Source: CAD feature listing. Evaluate the final solid. Frame: model axes, mm. Give positions to 0.01 mm unless a question says otherwise; leave off trailing zeros. Order: outer loops, then holes, each group sorted by start corner. A loop starts at its lowest first (then second) coordinate and runs counter-clockwise, first axis right, second up. Notation, with made-up numbers: M 84.5,-27 L 113.5,-27 A22 ccw 113.5,-6 Z; hole C 19.25,-34 d6. An arc over 180 degrees is marked long. Use CSV: the item, a comma, the result in double quotes. Start each with the question number.
Item 1: First-contact query: pin 1 (1 mm diameter, centred on x = -70, y = -2.5, fed in from +Z); pin 2 (1.2 mm diameter, centred on x = -100.5, y = -3, fed in from -Z). Flat tips, straight axial feed; report the tip coordinate or a pass-through.
Item 2: Ray query, probe 1 along Z at (x, y) = (-5, -1.45); probe 2 along Z at (x, y) = (47, -3.8); probe 3 along Z at (x, y) = (-62, -1.1). Return the intervals inside material, ascending. Write a range as from..to.
Item 3: Section query A-A on y = -3.1. Return loops of the section in (x, z), and give its area (3 significant figures).
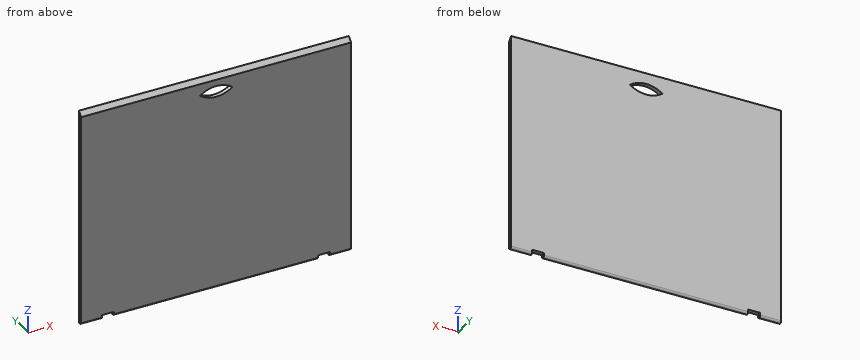
from build123d import *

# Parameters (mm, degrees)
F0_W     = 250
F0_H     = 197
F1_DEPTH = 4
F3_W     = 11
F3_H     = 4
F4_DEPTH = 0.5
F5_DEPTH = 250
F6_DEPTH = 25
F8_DEPTH = 25
F9_SIZE  = 3.99999


# Not quite as in the source:
# - a fillet or chamfer is up to 0.001 mm smaller than in the source, because OpenCascade refuses the exact size


with BuildPart() as f1:
    # F0 (on Front) → F1 (new body)
    with BuildSketch(Plane.XZ):
        Rectangle(F0_W, F0_H)
    extrude(amount=F1_DEPTH)

    # F3 (on face) → F4 (cut)
    with BuildSketch(Plane(origin=(0, 0, -98.5), x_dir=(1, 0, 0), z_dir=(0, 0, -1))):
        Polygon((-105.5, 0), (-94.5, 0), (-94.5, 4), (-105.5, 4), (-105.5, 2), align=None)
        with Locations((100, 2)):
            Rectangle(F3_W, F3_H)
    extrude(amount=-F4_DEPTH, mode=Mode.SUBTRACT)

    # F2 (on face) → F5 (join)
    with BuildSketch(Plane.YZ.offset(125)):
        with BuildLine():
            Line((-3.3228756555, -98.5), (-4, -98.5))
            Line((-4, -98.5), (-4, -100))
            ThreePointArc((-4, -100), (-3.8228756555, -99.1771243445), (-3.3228756555, -98.5))
        make_face()
        with BuildLine():
            ThreePointArc((-3.3228756555, -98.5), (-3.8228756555, -99.1771243445), (-4, -100))
            Line((-4, -100), (0, -100))
            ThreePointArc((0, -100), (-0.1771243445, -99.1771243445), (-0.6771243445, -98.5))
            Line((-0.6771243445, -98.5), (-3.3228756555, -98.5))
        make_face()
        with BuildLine():
            ThreePointArc((-0.6771243445, -98.5), (-0.1771243445, -99.1771243445), (0, -100))
            Line((0, -100), (0, -98.5))
            Line((0, -98.5), (-0.6771243445, -98.5))
        make_face()
        with BuildLine():
            Line((0, -100), (-4, -100))
            ThreePointArc((-4, -100), (-3.9878535848, -100.2200866318), (-3.9515618745, -100.4375))
            Line((-3.9515618745, -100.4375), (-2, -102))
            ThreePointArc((-2, -102), (-0.5857864376, -101.4142135624), (0, -100))
        make_face()
    extrude(amount=-F5_DEPTH)

    # F3 (on face) → F6 (cut)
    with BuildSketch(Plane(origin=(0, 0, -98.5), x_dir=(1, 0, 0), z_dir=(0, 0, -1))):
        Polygon((-105.5, 0), (-94.5, 0), (-94.5, 4), (-105.5, 4), (-105.5, 2), align=None)
        with Locations((100, 2)):
            Rectangle(F3_W, F3_H)
    extrude(amount=F6_DEPTH, mode=Mode.SUBTRACT)

    # F7 (on face) → F8 (cut)
    with BuildSketch(Plane.XZ.offset(4)):
        with BuildLine():
            ThreePointArc((-15, 83.5), (0, 78.4776194071), (15, 83.5))
            Line((15, 83.5), (5, 83.5))
            ThreePointArc((5, 83.5), (0, 78.5), (-5, 83.5))
            Line((-5, 83.5), (-15, 83.5))
        make_face()
        with BuildLine():
            Line((5, 83.5), (0, 83.5))
            Line((0, 83.5), (-5, 83.5))
            ThreePointArc((-5, 83.5), (0, 78.5), (5, 83.5))
        make_face()
        with BuildLine():
            Line((0, 83.5), (0, 88.5))
            ThreePointArc((0, 88.5), (-3.5355339059, 87.0355339059), (-5, 83.5))
            Line((-5, 83.5), (0, 83.5))
        make_face()
        with BuildLine():
            Line((0, 88.5), (0, 88.5776101571))
            ThreePointArc((0, 88.5776101571), (-7.918050974, 87.2737885484), (-15, 83.5))
            Line((-15, 83.5), (-5, 83.5))
            ThreePointArc((-5, 83.5), (-3.5355339059, 87.0355339059), (0, 88.5))
        make_face()
        with BuildLine():
            ThreePointArc((5, 83.5), (3.5355339059, 87.0355339059), (0, 88.5))
            Line((0, 88.5), (0, 83.5))
            Line((0, 83.5), (5, 83.5))
        make_face()
        with BuildLine():
            ThreePointArc((15, 83.5), (7.918050974, 87.2737885484), (0, 88.5776101571))
            Line((0, 88.5776101571), (0, 88.5))
            ThreePointArc((0, 88.5), (3.5355339059, 87.0355339059), (5, 83.5))
            Line((5, 83.5), (15, 83.5))
        make_face()
    extrude(amount=-F8_DEPTH, mode=Mode.SUBTRACT)

    # F9 (size 4 in the source; OpenCascade refuses exactly that, so slightly less here)
    f9_edges = [f1.edges().sort_by_distance(p)[0] for p in [
        (0, -4, 98.5),
    ]]
    chamfer(f9_edges, length=F9_SIZE)


solid = f1.part
Verdict:
1,pin 1,"z = 96.5"
1,pin 2,"z = -98"
2,probe 1,"-101.92..78.98, 88.07..97.05"
2,probe 2,"-100.56..94.7"
2,probe 3,"-101.79..97.4"
3,outline,"M -125,-101.12 L -105.5,-101.12 L -105.5,-98 L -94.5,-98 L -94.5,-101.12 L 94.5,-101.12 L 94.5,-98 L 105.5,-98 L 105.5,-101.12 L 125,-101.12 L 125,95.4 L -125,95.4 Z; hole M -15,83.5 A24.91 ccw 15,83.5 A24.69 ccw Z"
3,area,"48,900 mm2"
